Work out the finished part from the listing and answer in its coordinate system (mm). Round coordinates to 2 decimals unless told otherwise and drop trailing zeros. Write each loop counter-clockwise with the first axis right and the second up, starting at its lowest first coordinate (ties: lowest second). Pieces come first, ordered by that corner, then holes. Notation, with made-up numbers: (68, 57) -> (84, 57) arc R26 ccw to (84, 84) -> close; hole circle Ø10 at (61.5, 64.25). An arc over 180 degrees is marked (long way). Answer as a JSON object with one key per item and string values. Group by question number.
from build123d import *

# Parameters (mm, degrees)
EXTRUDE_1_DEPTH = 4


with BuildPart() as part:
    # Sketch 1 → Бобышка-Вытянуть1 (new body)
    with BuildSketch(Plane(origin=(-80.845718526, 0, 24.821686241), x_dir=(0.9308571955160213, 0, -0.36538319823994075), z_dir=(0, -1, 0))):
        Polygon((0, 0), (99.60171992, 39.096002212), (114.947814246, 0), (15.346094326, -39.096002212), (11.457373145, -37.39958022), (-1.696421992, -3.888721181), align=None)
        Polygon((15.380892726, -33.710949838), (28.412893463, -28.595585062), (23.297528688, -15.563584325), (10.265527951, -20.6789491), align=None, mode=Mode.SUBTRACT)
        Polygon((8.803995158, -16.955520318), (21.835995895, -11.840155543), (16.720631119, 1.191845194), (3.688630382, -3.923519581), align=None, mode=Mode.SUBTRACT)
        Polygon((19.513202706, 2.287994789), (24.628567481, -10.744005948), (37.660568219, -5.628641173), (32.545203443, 7.403359564), align=None, mode=Mode.SUBTRACT)
        Polygon((35.33777503, 8.499509159), (40.453139805, -4.532491578), (53.485140542, 0.582873197), (48.369775767, 13.614873934), align=None, mode=Mode.SUBTRACT)
        Polygon((51.162347354, 14.711023529), (64.194348091, 19.826388304), (69.309712866, 6.794387567), (56.277712129, 1.679022792), align=None, mode=Mode.SUBTRACT)
        Polygon((95.843492738, 32.249417045), (100.958857514, 19.217416307), (87.926856776, 14.102051532), (82.811492001, 27.134052269), align=None, mode=Mode.SUBTRACT)
        Polygon((66.986919677, 20.922537899), (80.018920415, 26.037902675), (85.13428519, 13.005901937), (72.102284453, 7.890537162), align=None, mode=Mode.SUBTRACT)
        Polygon((73.559385355, 4.17839915), (86.591386092, 9.293763925), (91.711182758, -3.749527582), (78.679182021, -8.864892357), align=None, mode=Mode.SUBTRACT)
        Polygon((89.383957678, 10.38991352), (94.503754345, -2.653377987), (107.535755082, 2.461986788), (102.415958416, 15.505278295), align=None, mode=Mode.SUBTRACT)
        Polygon((70.766813768, 3.082249555), (75.886610434, -9.961041952), (62.854609697, -15.076406727), (57.734813031, -2.03311522), align=None, mode=Mode.SUBTRACT)
        Polygon((54.942241444, -3.129264815), (60.062038111, -16.172556322), (47.030037373, -21.287921097), (41.910240707, -8.24462959), align=None, mode=Mode.SUBTRACT)
        Polygon((39.117669121, -9.340779185), (44.237465787, -22.384070692), (31.20546505, -27.499435468), (26.085668383, -14.456143961), align=None, mode=Mode.SUBTRACT)
    extrude(amount=-EXTRUDE_1_DEPTH)


solid = part.part
1) This flat-tipped pin is pushed along its axis until it touches: P1, Ø5, axis at x = -22, z = -9.5, coming from the -Y side (3 decimals). Where does it stop, or does it pass through?
2) A cutting plane is placed at B-B on z = 9. Determine the outline of the cut face in (x, y).
3) A cutting plane is placed at C-C on y = 1.55. State how many separate pieces and enclosed holes the cut face has, plus the area to 3 significant figures.
4) A cutting plane is placed at D-D on x = -8.5. Determine the outline of the cut face in (y, z).
5) Straight lines are drawn through the part: L1, parallel to Z at x = -8.5, y = 3.7; L2, parallel to X at y = 1.55, z = 22.5; L3, parallel to X at y = 1.05, z = 23.5. For each, find the intervals that lie inside material, in ascending order.
6) For a pull along Z with two mould halves and no side action, classify faces 1 (the face through (-83.846, 2, 4)), 2 (the face through (-21, 2, -12.178)), 3 (the face through (-82.37, 1.97, 23.3)) as released by +Z, released by -Z, zero draft, split by the parting line, or undercut.
7) A cutting plane is placed at A-A on x = -76. Determine the outline of the cut face in (y, z).
Established:
{
 "1": {"P1": "passes through"},
 "2": {"outline": "(-83.85, 0) -> (-78.85, 0) -> (-78.85, 4) -> (-83.85, 4) -> close; (-64.85, 0) -> (-61.85, 0) -> (-61.85, 4) -> (-64.85, 4) -> close; (-47.85, 0) -> (-44.85, 0) -> (-44.85, 4) -> (-47.85, 4) -> close; (-30.85, 0) -> (-27.85, 0) -> (-27.85, 4) -> (-30.85, 4) -> close; (-13.85, 0) -> (-10.85, 0) -> (-10.85, 4) -> (-13.85, 4) -> close; (3.15, 0) -> (6.15, 0) -> (6.15, 4) -> (3.15, 4) -> close; (20.15, 0) -> (26.15, 0) -> (26.15, 4) -> (20.15, 4) -> close"},
 "3": {"separate pieces": "1", "enclosed holes": "12", "area": "2,260 mm²"},
 "4": {"outline": "(0, -17.18) -> (4, -17.18) -> (4, -12.18) -> (0, -12.18) -> close; (0, 1.83) -> (4, 1.83) -> (4, 5.82) -> (0, 5.82) -> close; (0, 19.82) -> (4, 19.82) -> (4, 24.82) -> (0, 24.82) -> close"},
 "5": {"L1": "z = -17.18 to -12.18, 1.83 to 5.82, 19.82 to 24.82", "L2": "x = -83.17 to 26.15", "L3": "x = -82.17 to 26.15"},
 "6": {"face 1": "zero draft", "face 2": "undercut", "face 3": "released by +Z"},
 "7": {"outline": "(0, -17.18) -> (4, -17.18) -> (4, -12.18) -> (0, -12.18) -> close; (0, 1.82) -> (4, 1.82) -> (4, 5.82) -> (0, 5.82) -> close; (0, 19.82) -> (4, 19.82) -> (4, 24.82) -> (0, 24.82) -> close"}
}
